Can you work these out from the model? Positions are in its coordinate system, mm. Round coordinates to 2 decimals unless told otherwise and drop trailing zeros. Loops run counter-clockwise (first coordinate to the right, second up) from the corner with the lowest first, then second, coordinate; pieces in that order, holes last.
Autodesk Inventor part; units mm, degrees
ref_plane "YZ Plane" through (0, 0, 0) normal (1, 0, 0) x (0, 1, 0)
ref_plane "XZ Plane" through (0, 0, 0) normal (0, 1, 0) x (-1, 0, 0)
ref_plane "XY Plane" through (0, 0, 0) normal (0, 0, 1) x (1, 0, 0)
sketch "Sketch1" plane through (0, 0, 0) normal (0, 0, 1) x (1, 0, 0)
  line L0 (0, 0) -> (419.1, 0)
  line L1 (419.1, 0) -> (419.1, 254)
  line L2 (419.1, 254) -> (0, 254)
  line L3 (0, 254) -> (0, 0)
  line L4 (273.05, 184.15) -> (349.25, 184.15)
  line L5 (349.25, 184.15) -> (349.25, 0)
  line L6 (349.25, 0) -> (273.05, 0)
  line L7 (273.05, 0) -> (273.05, 184.15)
  circle A0 centre (76.2, 88.9) radius 12.7
  line L8 (63.5, 88.9) -> (88.9, 88.9)
  line L9 (88.9, 88.9) -> (88.9, 0)
  line L10 (88.9, 0) -> (63.5, 0)
  line L11 (63.5, 0) -> (63.5, 88.9)
  dimension "d5" = 25.4
  dimension "d0" = 419.1
  dimension "d1" = 254
  dimension "d2" = 76.2
  dimension "d3" = 184.15
  dimension "d4" = 273.05
  dimension "d6" = 88.9
  dimension "d7" = 63.5
  dimension "d8" = 25.4
  dimension "d9" = 76.2
extrude "Extrusion1" add sketch "Sketch1" along normal mid plane 12.7 contours L3 L2 L1 L0 L5 L4 L7 L9 A0 L11
fillet "Fillet1" radius 3.175 1 edges at (273.05, 184.15, 0)
fillet "Fillet2" radius 3.175 1 edges at (349.25, 184.15, 0)
equation "\"d0\" = Length"
equation "\"d1\" = Height"
equation "\"d10\" = Thick"
properties part number "InsideWall"
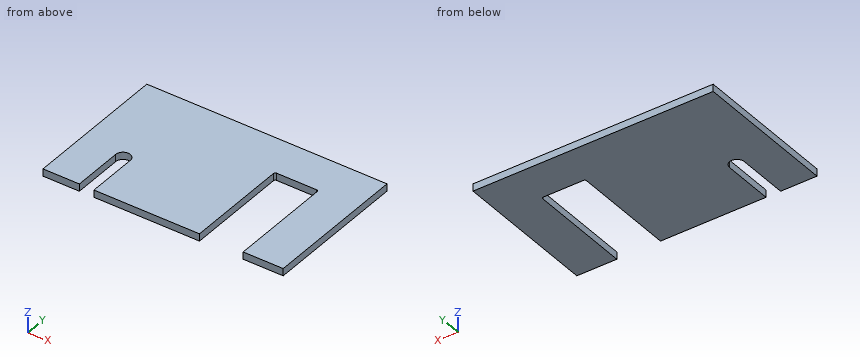
(1) If we section it at C-C, the plane x = 76.2: List the corners of the cut face in (y, z) for me, then the cut area to 3 significant figures.
Worked answers:
outline: (101.6, -6.35) - (254, -6.35) - (254, 6.35) - (101.6, 6.35) - close
area: 1,940 mm2
(2) If I drill on line 1 (X direction, y = 73.5, z = 1); line 2 (X direction, y = 164, z = 5.75); line 3 (X direction, y = 98, z = 1), over which ranges is the centre line in solid material (lowest first)?
Worked answers:
line 1: x = 0 to 63.5, 88.9 to 273.05, 349.25 to 419.1
line 2: x = 0 to 273.05, 349.25 to 419.1
line 3: x = 0 to 67.34, 85.06 to 273.05, 349.25 to 419.1
(3) If we section it at B-B, the plane z = 1.5: List the corners of the cut face in (x, y) for me (3 decimals).
Worked answers:
outline: (0, 0) - (63.5, 0) - (63.5, 88.9) arc R12.7 cw to (88.9, 88.9) - (88.9, 0) - (273.05, 0) - (273.05, 180.975) arc R3.175 cw to (276.225, 184.15) - (346.075, 184.15) arc R3.175 cw to (349.25, 180.975) - (349.25, 0) - (419.1, 0) - (419.1, 254) - (0, 254) - close
(4) Will these pins go through, and if not, where does the flat tip stop? P1, Ø4, axis at x = 308.5, z = -2.5, coming from the -Y side; P2, Ø6.5, axis at y = 119, z = 0.5, coming from the -X side.
Worked answers:
P1: stops at y = 184.15
P2: stops at x = 0
(5) If we section it at A-A, the plane y = 42.5: List the corners of the cut face in (x, z) for me, then the cut area to 3 significant figures.
Worked answers:
outline: (0, -6.35) - (63.5, -6.35) - (63.5, 6.35) - (0, 6.35) - close; (88.9, -6.35) - (273.05, -6.35) - (273.05, 6.35) - (88.9, 6.35) - close; (349.25, -6.35) - (419.1, -6.35) - (419.1, 6.35) - (349.25, 6.35) - close
area: 4,030 mm2
